Can you work these out from the model? Positions are in its coordinate system, mm. A direction names the side the tool comes from. Give positions to 0.01 mm unless a question says otherwise; leave off trailing zeros. Order: outer loops, then holes, each group sorted by start corner. A loop starts at its lowest first (then second) coordinate and runs counter-clockwise, first axis right, second up. Notation, with made-up numbers: M 25.25,75 L 36.25,75 A17 ccw 36.25,89 Z; hole C -11,46.25 d8. An arc over 180 degrees is marked long. Write each question's results on one line, items separated by ' | '.
from build123d import *

# Parameters (mm, degrees)
CROQUIS1_W              = 22.5
CROQUIS1_H              = 12.5
SALIENTE_EXTRUIR1_DEPTH = 22.5
CROQUIS2_W              = 5
CROQUIS2_H              = 2.5
SALIENTE_EXTRUIR2_DEPTH = 12.5
CORTAR_EXTRUIR1_REACH   = 27.404
CROQUIS3_R              = 1
CROQUIS4_R              = 6.25
SALIENTE_EXTRUIR3_DEPTH = 4.5
CROQUIS5_R              = 2.5
SALIENTE_EXTRUIR4_DEPTH = 3


with BuildPart() as part:
    # Croquis1 → Saliente-Extruir1 (new body)
    with BuildSketch(Plane(origin=(0, 0, 0), x_dir=(1, 0, 0), z_dir=(0, 1, 0))):
        Rectangle(CROQUIS1_W, CROQUIS1_H)
    extrude(amount=SALIENTE_EXTRUIR1_DEPTH)

    # Croquis2 → Saliente-Extruir2 (add)
    with BuildSketch(Plane.XY.offset(6.25)):
        with Locations((13.75, 17.25)):
            Rectangle(CROQUIS2_W, CROQUIS2_H)
        with Locations((-13.75, 17.25)):
            Rectangle(CROQUIS2_W, CROQUIS2_H)
    extrude(amount=-SALIENTE_EXTRUIR2_DEPTH)

    # Croquis3 → Cortar-Extruir1 (cut, up to next)
    with BuildSketch(Plane(origin=(0, 18.5, 0), x_dir=(1, 0, 0), z_dir=(0, 1, 0)), mode=Mode.PRIVATE) as cortar_extruir1_sk1:
        with Locations(Location((13.75, 0, 0), (0, 0, 270))):
            Circle(CROQUIS3_R)
    cortar_extruir1_tool1 = extrude(cortar_extruir1_sk1.sketch, amount=-CORTAR_EXTRUIR1_REACH, mode=Mode.PRIVATE) & part.part
    # Croquis3 → Cortar-Extruir1 (cut, up to next)
    with BuildSketch(Plane(origin=(0, 18.5, 0), x_dir=(1, 0, 0), z_dir=(0, 1, 0)), mode=Mode.PRIVATE) as cortar_extruir1_sk2:
        with Locations(Location((-13.75, 0, 0), (0, 0, 270))):
            Circle(CROQUIS3_R)
    cortar_extruir1_tool2 = extrude(cortar_extruir1_sk2.sketch, amount=-CORTAR_EXTRUIR1_REACH, mode=Mode.PRIVATE) & part.part
    add(cortar_extruir1_tool1.solids().sort_by_distance((13.75, 18.5, 0))[0], mode=Mode.SUBTRACT)
    add(cortar_extruir1_tool2.solids().sort_by_distance((-13.75, 18.5, 0))[0], mode=Mode.SUBTRACT)

    # Croquis4 → Saliente-Extruir3 (add)
    with BuildSketch(Plane(origin=(0, 22.5, 0), x_dir=(1, 0, 0), z_dir=(0, 1, 0))):
        with Locations(Location((5, 0, 0), (0, 0, 270))):
            Circle(CROQUIS4_R)
    extrude(amount=SALIENTE_EXTRUIR3_DEPTH)

    # Croquis5 → Saliente-Extruir4 (add)
    with BuildSketch(Plane(origin=(0, 27, 0), x_dir=(1, 0, 0), z_dir=(0, 1, 0))):
        with Locations(Location((5.218378147, 0, 0), (0, 0, 270))):
            Circle(CROQUIS5_R)
    extrude(amount=SALIENTE_EXTRUIR4_DEPTH)


solid = part.part
(1) Imagine slicing it at B-B, the plane y = 18. Write out the boundary of the cut face in (x, z).
Data:
outline: M -16.25,-6.25 L 16.25,-6.25 L 16.25,6.25 L -16.25,6.25 Z; hole C -13.75,0 d2; hole C 13.75,0 d2
(2) I need wall thicknesses on L1, parallel to X at y = 16.75, z = 0; L2, parallel to X at y = 12.5, z = -5.25; L3, parallel to Y at x = -3, z = 5.25. Which ranges of each line are inside material? Lowest first, please. Write a range as from..to.
Data:
L1: x = -16.25..-14.75, -12.75..12.75, 14.75..16.25 | L2: x = -11.25..11.25 | L3: y = 0..22.5
(3) Will these pins go through, and if not, where does the flat tip stop? P1, Ø2.5, axis at x = -13.75, z = 0, coming from the +Y side; P2, Ø4, axis at x = 0, z = 1.5, coming from the +Y side; P3, Ø2, axis at y = 11.5, z = 1, coming from the -X side.
Data:
P1: stops at y = 18.5 | P2: stops at y = 27 | P3: stops at x = -11.25
(4) For faces 1 (the face through (2, 27, 0)), 2 (the face through (15, 18.5, 0)), 3 (the face through (-11.25, 8, 0)), which set-ups out of +Z, -Z, +X, -X, +Y, -Y let a thin tool reach every point of the face, with its end or its side?
Data:
face 1: +Y | face 2: +Z, -Z, +X, +Y | face 3: +Z, -Z, -X, -Y
(5) Imagine slicing it at A-A, the plane x = -13.75. Write out the boundary of the cut face in (y, z), plus the area to 4 significant figures.
Data:
outline: M 16,-6.25 L 18.5,-6.25 L 18.5,-1 L 16,-1 Z; M 16,1 L 18.5,1 L 18.5,6.25 L 16,6.25 Z | area: 26.25 mm2
(6) We'd pull the mould along X, two halves only. Please class faces 4 (the face through (12.774, 17.268, -0.217)), 5 (the face through (10, 22.5, -5)), 6 (the face through (7.33, 28.48, 1.34)): +X half, -X half, draft (parallel to the pull), parting line (faces both ways), or undercut.
Data:
face 4: undercut | face 5: draft | face 6: parting line
(7) Imagine slicing it at C-C, the plane x = 10. Write out the boundary of the cut face in (y, z).
Data:
outline: M 0,-6.25 L 22.5,-6.25 L 22.5,-3.75 L 27,-3.75 L 27,3.75 L 22.5,3.75 L 22.5,6.25 L 0,6.25 Z
(8) Imagine slicing it at D-D, the plane y = 9. Write out the boundary of the cut face in (x, z).
Data:
outline: M -11.25,-6.25 L 11.25,-6.25 L 11.25,6.25 L -11.25,6.25 Z
